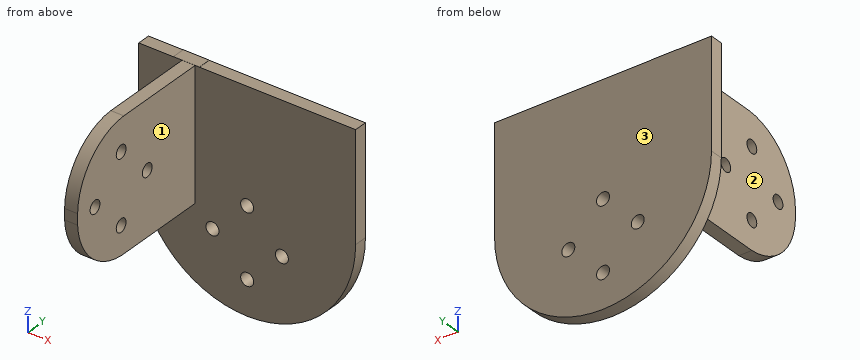
from build123d import *

# Parameters (mm, degrees)
BOSS_EXTRU_1_DEPTH      = 3
ESQUISSE4_W             = 4
ESQUISSE4_H             = 25
ENL_V_MAT_EXTRU_1_DEPTH = 3
ESQUISSE5_R             = 1.5
ENL_V_MAT_EXTRU_2_DEPTH = 3
ESQUISSE9_W             = 25.088970056
ESQUISSE9_H             = 3
BOSS_EXTRU_5_DEPTH      = 6
ESQUISSE10_W            = 3
ESQUISSE10_H            = 30
BOSS_EXTRU_6_DEPTH      = 36
ESQUISSE12_R            = 1.5
ENL_V_MAT_EXTRU_3_DEPTH = 36
ESQUISSE8_W             = 25.033293463
ESQUISSE8_H             = 3
BOSS_EXTRU_4_DEPTH      = 6


with BuildPart() as part:
    # Esquisse2 → Boss.-Extru.1 (new body)
    with BuildSketch(Plane(origin=(0, 0, 0), x_dir=(1, 0, 0), z_dir=(0, 1, 0))):
        with BuildLine():
            Line((-25, 0), (-25, -25))
            Line((-25, -25), (25, -25))
            Line((25, -25), (25, 0))
            ThreePointArc((25, 0), (0, 25), (-25, 0))
        make_face()
    extrude(amount=BOSS_EXTRU_1_DEPTH)

    # Esquisse4 → Enlèv. mat.-Extru.1 (cut)
    with BuildSketch(Plane.XZ):
        with Locations((-13, 12.5)):
            Rectangle(ESQUISSE4_W, ESQUISSE4_H)
    extrude(amount=-ENL_V_MAT_EXTRU_1_DEPTH, mode=Mode.SUBTRACT)

    # Esquisse5 → Enlèv. mat.-Extru.2 (cut)
    with BuildSketch(Plane.XZ):
        with Locations(Location((8, -9, 0), (0, 0, 270))):
            Circle(ESQUISSE5_R)
        with Locations(Location((-8, -9, 0), (0, 0, 270))):
            Circle(ESQUISSE5_R)
        with Locations(Location((0, -17, 0), (0, 0, 270))):
            Circle(ESQUISSE5_R)
        with Locations(Location((0, -1, 0), (0, 0, 270))):
            Circle(ESQUISSE5_R)
    extrude(amount=-ENL_V_MAT_EXTRU_2_DEPTH, mode=Mode.SUBTRACT)

    # Esquisse9 → Boss.-Extru.5 (add)
    with BuildSketch(Plane(origin=(-15, 0, 0), x_dir=(0, 0, -1), z_dir=(1, 0, 0))):
        with Locations((-12.455514972, 1.5)):
            Rectangle(ESQUISSE9_W, ESQUISSE9_H)
    extrude(amount=BOSS_EXTRU_5_DEPTH)

    # Esquisse10 → Boss.-Extru.6 (add)
    with BuildSketch(Plane.XZ):
        with Locations((-13.5, 10)):
            Rectangle(ESQUISSE10_W, ESQUISSE10_H)
    extrude(amount=BOSS_EXTRU_6_DEPTH)

    # Esquisse12 → Enlèv. mat.-Extru.3 (cut)
    with BuildSketch(Plane(origin=(-12, 0, 0), x_dir=(0, 0, 1), z_dir=(1, 0, 0))):
        with BuildLine():
            Line((-5, 36), (-5, 22.662353219))
            ThreePointArc((-5, 22.662353219), (-0.867271737, 31.867271737), (8.337646782, 36))
            Line((8.337646782, 36), (-5, 36))
        make_face()
        with BuildLine():
            Line((25, 36), (10.831176607, 36))
            ThreePointArc((10.831176607, 36), (20.732510765, 31.732510766), (25, 21.831176609))
            Line((25, 21.831176609), (25, 36))
        make_face()
        with Locations(Location((9.585618663, 30.662353219, 0), (0, 0, 180))):
            Circle(ESQUISSE12_R)
        with Locations(Location((1.585618663, 22.662353219, 0), (0, 0, 180))):
            Circle(ESQUISSE12_R)
        with Locations(Location((9.585618663, 14.662353219, 0), (0, 0, 180))):
            Circle(ESQUISSE12_R)
        with Locations(Location((17.585618663, 22.662353219, 0), (0, 0, 180))):
            Circle(ESQUISSE12_R)
    extrude(amount=-ENL_V_MAT_EXTRU_3_DEPTH, mode=Mode.SUBTRACT)

    # Esquisse8 → Boss.-Extru.4 (add)
    with BuildSketch(Plane.ZY.offset(11)):
        with Locations((12.516646732, 1.5)):
            Rectangle(ESQUISSE8_W, ESQUISSE8_H)
    extrude(amount=BOSS_EXTRU_4_DEPTH)


solid = part.part
Input: part model. Units: mm. Frame: model coordinates. Face numbers are marked on the shaded views. A direction names the side the tool comes from. Give positions to 0.01 mm unless a question says otherwise; leave off trailing zeros. Write each loop counter-clockwise with the first axis right and the second up, starting at its lowest first coordinate (ties: lowest second). Pieces come first, ordered by that corner, then holes.
Q1. Set-up query: the marked faces 1, 2 and 3. Return all of +Z, -Z, +X, -X, +Y, -Y with unobstructed straight access to the full face (end or side cutting, diameter ignored); none if empty.
Q2. Section C-C, the plane x = -13. State how many separate pieces and enclosed holes the cut face has, plus the area to 3 significant figures.
Q3. Material intervals for probe 1 along X at (y, z) = (1, -9); probe 2 along Z at (x, y) = (-14, -17); probe 3 along X at (y, z) = (-20, 5), sorted ascending.
Q4. Section D-D, the plane y = -6. Output: boundary loops of the cut face in (x, z), plus the area to 3 significant figures.
Q5. Section B-B, the plane z = -1. Output: boundary loops of the cut face in (x, y).
Q6. Section A-A, the plane x = 0. Output: boundary loops of the cut face in (y, z).
Q7. First-contact query: P1, Ø1.8, axis at x = 0, z = -1, coming from the -Y side; P2, Ø2.5, axis at x = -13, y = -9, coming from the +Z side; P3, Ø1.5, axis at x = -13, y = -15, coming from the -Z side; P4, Ø6, axis at x = 13.5, z = 2, coming from the -Y side. Flat tips, straight axial feed; report the tip coordinate or a pass-through.
Filled in:
1. face 1: +Z, -Z, +X, -Y
1. face 2: +Z, -Z, -X, -Y
1. face 3: +Z, -Z, +X, -X, +Y
2. separate pieces: 1
2. enclosed holes: 4
2. area: 1,100 mm2
3. probe 1: x = -23.32 to -9.5, -6.5 to 6.5, 9.5 to 23.32
3. probe 2: z = -5 to 25
3. probe 3: x = -15 to -12
4. outline: (-15, -5) - (-12, -5) - (-12, 25) - (-15, 25) - close
4. area: 90.0 mm2
5. outline: (-24.98, 0) - (-15, 0) - (-15, -31.73) - (-12, -31.73) - (-12, 0) - (-1.5, 0) - (-1.5, 3) - (-24.98, 3) - close; (1.5, 0) - (24.98, 0) - (24.98, 3) - (1.5, 3) - close
6. outline: (0, -25) - (3, -25) - (3, -18.5) - (0, -18.5) - close; (0, -15.5) - (3, -15.5) - (3, -2.5) - (0, -2.5) - close; (0, 0.5) - (3, 0.5) - (3, 25) - (0, 25) - close
7. P1: passes through
7. P2: stops at z = 25
7. P3: stops at z = -5
7. P4: stops at y = 0
